Read the model definition and answer for the solid it produces. Units are mm, in the model's axes. Give positions to 0.01 mm unless a question says otherwise; leave off trailing zeros. One line per item, written item: value. Start each with the question number.
```python
from build123d import *

# Parameters (mm, degrees)
F0_W     = 70
F0_H     = 105
F0_R     = 1
F1_DEPTH = 3.175


with BuildPart() as f1:
    # F0 (on Front) → F1 (new body)
    with BuildSketch(Plane.XZ):
        Rectangle(F0_W, F0_H)
        with Locations((-30, -47.5)):
            Circle(F0_R, mode=Mode.SUBTRACT)
        with Locations((-30, -27.5)):
            Circle(F0_R, mode=Mode.SUBTRACT)
        with Locations((-15, -47.5)):
            Circle(F0_R, mode=Mode.SUBTRACT)
        with Locations((-15, -27.5)):
            Circle(F0_R, mode=Mode.SUBTRACT)
        with Locations((15, -47.5)):
            Circle(F0_R, mode=Mode.SUBTRACT)
        with Locations((15, -27.5)):
            Circle(F0_R, mode=Mode.SUBTRACT)
        with Locations((30, -47.5)):
            Circle(F0_R, mode=Mode.SUBTRACT)
        with Locations((30, -27.5)):
            Circle(F0_R, mode=Mode.SUBTRACT)
        with Locations((-30, 27.5)):
            Circle(F0_R, mode=Mode.SUBTRACT)
        with Locations((-30, 47.5)):
            Circle(F0_R, mode=Mode.SUBTRACT)
        with Locations((-15, 27.5)):
            Circle(F0_R, mode=Mode.SUBTRACT)
        with Locations((-15, 47.5)):
            Circle(F0_R, mode=Mode.SUBTRACT)
        with Locations((15, 27.5)):
            Circle(F0_R, mode=Mode.SUBTRACT)
        with Locations((15, 47.5)):
            Circle(F0_R, mode=Mode.SUBTRACT)
        with Locations((30, 27.5)):
            Circle(F0_R, mode=Mode.SUBTRACT)
        with Locations((30, 47.5)):
            Circle(F0_R, mode=Mode.SUBTRACT)
    extrude(amount=F1_DEPTH)


solid = f1.part
```
1) The mould has two halves that part along X. Classify faces 1 (the flat face through (-35, -2, -1)), 2 (the flat face through (0, -2, -52.5)), 3 (the cylindrical face through (29.87, -1.57, -26.51)): +X half, -X half, draft (parallel to the pull), parting line (faces both ways), or undercut.
2) Find the intervals of material crossed by probe 1 along Z at (x, y) = (30, -1.3); probe 2 along Z at (x, y) = (29.5, -0.65), in increasing order. Write a range as from..to.
3) This flat-tipped pin is pushed along its axis until it touches: pin 1 (1.6 mm diameter, centred on x = -30, z = 27.5, fed in from +Y). Where does it stop, or does it pass through?
Solved:
1. face 1: -X half
1. face 2: draft
1. face 3: undercut
2. probe 1: z = -52.5..-48.5, -46.5..-28.5, -26.5..26.5, 28.5..46.5, 48.5..52.5
2. probe 2: z = -52.5..-48.37, -46.63..-28.37, -26.63..26.63, 28.37..46.63, 48.37..52.5
3. pin 1: passes through
